For this review, take the finished solid that the model builds, in its own axes (mm). Give positions to 0.01 mm unless a question says otherwise; leave off trailing zeros. Order: outer loops, then holes, each group sorted by start corner. A loop starts at its lowest first (then second) coordinate and runs counter-clockwise, first axis right, second up. Notation, with made-up numbers: (-7.75, 15.5) - (30.25, 15.5) arc R14 ccw to (30.25, 32.5) - close; hole circle Ø4 at (-4.75, -1). An arc over 180 degrees is marked (long way). One line per item, written item: value.
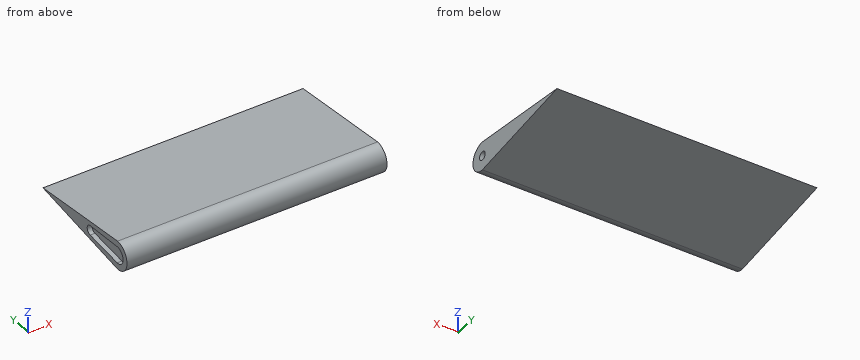
```python
from build123d import *

# Parameters (mm, degrees)
F0_R     = 2.8575
F1_DEPTH = 114.3
F2_DEPTH = 2.0828
F3_R     = 1.905
F4_DEPTH = 25.4


with BuildPart() as f1:
    # F0 (on Right) → F1 (new body)
    with BuildSketch(Plane.YZ):
        with BuildLine():
            Line((50.401562, 0), (0, 6.35))
            ThreePointArc((0, 6.35), (-6.35, 0), (0, -6.35))
            Line((0, -6.35), (50.401562, 0))
        make_face()
        with BuildLine():
            ThreePointArc((0.305643, -3.670296), (-3.683, 0), (0.305643, 3.670296))
            Line((0.305643, 3.670296), (18.54337, 2.151553))
            ThreePointArc((18.54337, 2.151553), (20.5232, 0), (18.54337, -2.151553))
            Line((18.54337, -2.151553), (0.305643, -3.670296))
        make_face(mode=Mode.SUBTRACT)
        with BuildLine():
            Line((18.54337, 2.151553), (0.305643, 3.670296))
            ThreePointArc((0.305643, 3.670296), (-3.683, 0), (0.305643, -3.670296))
            Line((0.305643, -3.670296), (18.54337, -2.151553))
            ThreePointArc((18.54337, -2.151553), (20.5232, 0), (18.54337, 2.151553))
        make_face()
        Circle(F0_R, mode=Mode.SUBTRACT)
        Circle(F0_R)
    extrude(amount=F1_DEPTH)

    # F0 (on Right) → F2 (cut)
    with BuildSketch(Plane.YZ):
        with BuildLine():
            Line((18.54337, 2.151553), (0.305643, 3.670296))
            ThreePointArc((0.305643, 3.670296), (-3.683, 0), (0.305643, -3.670296))
            Line((0.305643, -3.670296), (18.54337, -2.151553))
            ThreePointArc((18.54337, -2.151553), (20.5232, 0), (18.54337, 2.151553))
        make_face()
        Circle(F0_R, mode=Mode.SUBTRACT)
        Circle(F0_R)
    extrude(amount=F2_DEPTH, mode=Mode.SUBTRACT)

    # F3 (on face) → F4 (cut)
    with BuildSketch(Plane.YZ.offset(114.3)):
        Circle(F3_R)
    extrude(amount=-F4_DEPTH, mode=Mode.SUBTRACT)


solid = f1.part
```
(1) Take a section at D-D (y = 15.5). Write out the cut boundary in (x, z), then the cut area to 3 significant figures.
Answers below:
outline: (0, -4.4) - (114.3, -4.4) - (114.3, 4.4) - (0, 4.4) - (0, 2.4) - (2.08, 2.4) - (2.08, -2.4) - (0, -2.4) - close
area: 995 mm^2
(2) Wall thickness on line 1 (Z direction, x = 1, y = 0); line 2 (Z direction, x = 105, y = 0) (3 decimals); line 3 (X direction, y = 5.5, z = -1.5): over which ranges is each line inside the solid? List them lowest first. Write a range as from..to.
Answers below:
line 1: z = -6.35..-3.68, 3.68..6.35
line 2: z = -6.35..-1.905, 1.905..6.35
line 3: x = 2.08..114.3
(3) For P1, Ø6, axis at x = 53.5, y = 12, coming from the +Z side; P2, Ø2, axis at x = 40.5, z = 2.5, coming from the -Y side; P3, Ø1, axis at y = 24.5, z = 4, coming from the -X side; P4, Ø3.5, axis at y = 7, z = 0, coming from the -X side, all flat-tipped, find the tip position at first contact; note any pin that passes through.
Answers below:
P1: stops at z = 5.22
P2: stops at y = -6.17
P3: passes through
P4: stops at x = 2.08
(4) Take a section at A-A (y = 4). Write out the cut boundary in (x, z).
Answers below:
outline: (0, -5.85) - (114.3, -5.85) - (114.3, 5.85) - (0, 5.85) - (0, 3.36) - (2.08, 3.36) - (2.08, -3.36) - (0, -3.36) - close
(5) Take a section at C-C (z = -5). Write out the cut boundary in (x, y), then the cut area to 3 significant figures.
Answers below:
outline: (0, -3.91) - (114.3, -3.91) - (114.3, 10.72) - (0, 10.72) - close
area: 1,670 mm^2
(6) Take a section at B-B (x = 47). Write out the cut boundary in (y, z), then the cut area to 3 significant figures.
Answers below:
outline: (0, -6.35) - (50.4, 0) - (0, 6.35) arc R6.35 ccw to start
area: 383 mm^2
